```python
from build123d import *

# Parameters (mm, degrees)
F0_W     = 5
F0_H     = 7.5
F2_DEPTH = 39
F3_W     = 41.4538450539
F3_H     = 32
F4_DEPTH = 50
F5_R     = 7.5
F6_DEPTH = 78.001


with BuildPart() as f1:
    # F0 (on Front) → F1 (revolve)
    with BuildSketch(Plane.XZ):
        Polygon((5, 7.5), (5, 0), (19, 0), (19, 3), (35, 3), (35, 7.5), align=None)
        with Locations((2.5, 3.75)):
            Rectangle(F0_W, F0_H)
        Polygon((0, 20), (0, 7.5), (5, 7.5), (5, 30), (0, 30), align=None)
    revolve(axis=Axis((17.5, 0, 0), (1, 0, 0)))

    # F0 (on Front) → F2 (join, symmetric)
    with BuildSketch(Plane.XZ):
        with BuildLine():
            ThreePointArc((-30, -20), (-15.8578643763, -14.1421356237), (-10, 0))
            ThreePointArc((-10, 0), (-15.8578643763, 14.1421356237), (-30, 20))
            ThreePointArc((-30, 20), (-50, 0), (-30, -20))
        make_face()
        with BuildLine():
            Line((-10, 0), (0, 0))
            Line((0, 0), (0, 7.5))
            Line((0, 7.5), (0, 20))
            Line((0, 20), (-30, 20))
            ThreePointArc((-30, 20), (-15.8578643763, 14.1421356237), (-10, 0))
        make_face()
        with BuildLine():
            Line((0, -7.5), (0, 0))
            Line((0, 0), (-10, 0))
            ThreePointArc((-10, 0), (-15.8578643763, -14.1421356237), (-30, -20))
            Line((-30, -20), (0, -20))
            Line((0, -20), (0, -7.5))
        make_face()
    extrude(amount=F2_DEPTH, both=True)

    # F3 (on Top) → F4 (cut, symmetric)
    with BuildSketch(Plane.XY):
        with Locations((-29.273077473, -16)):
            Rectangle(F3_W, F3_H)
        with Locations((-29.273077473, 16)):
            Rectangle(F3_W, F3_H)
    extrude(amount=F4_DEPTH, both=True, mode=Mode.SUBTRACT)

    # F5 (on face) → F6 (cut, through all)
    with BuildSketch(Plane.XZ.offset(39)):
        with Locations((-30, 0)):
            Circle(F5_R)
    extrude(amount=-F6_DEPTH, mode=Mode.SUBTRACT)


solid = f1.part
```
Work out the finished part from the listing and answer in its coordinate system (mm). A direction names the side the tool comes from. Coordinates: 2 decimals unless noted, no trailing zeros. Loops run counter-clockwise (first coordinate to the right, second up) from the corner with the lowest first, then second, coordinate; pieces in that order, holes last. Notation, with made-up numbers: (78.5, 17) -> (132.5, 17) arc R13 ccw to (132.5, 40) -> close; hole circle Ø5 at (-4.75, 85). An arc over 180 degrees is marked (long way). Answer as CSV lines item,"result".
Q1. The part is cut by section D-D on x = 30. Write down the section's boundary in (y, z), and give its area (3 significant figures).
Findings:
outline,"circle Ø15 at (0, 0); hole circle Ø6 at (0, 0)"
area,"148 mm²"
Q2. The part is cut by section A-A on z = 0. Write down the section's boundary in (x, y).
Findings:
outline,"(-50, -39) -> (-37.5, -39) -> (-37.5, -32) -> (-50, -32) -> close; (-50, 32) -> (-37.5, 32) -> (-37.5, 39) -> (-50, 39) -> close; (-22.5, -39) -> (0, -39) -> (0, -30) -> (5, -30) -> (5, -7.5) -> (35, -7.5) -> (35, -3) -> (19, -3) -> (19, 3) -> (35, 3) -> (35, 7.5) -> (5, 7.5) -> (5, 30) -> (0, 30) -> (0, 39) -> (-22.5, 39) -> (-22.5, 32) -> (-8.55, 32) -> (-8.55, -32) -> (-22.5, -32) -> close"
Q3. A tool of negligible diameter and unlimited length cuts with its end or side. For faces 1 (the face through (-5, -1, -20)), 2 (the face through (-8.546, 0, 0)), 3 (the face through (19.79, -0.33, -7.493)), from which of +Z, -Z, +X, -X, +Y, -Y can it reach the whole face along a straight path? Write none if from no direction.
Findings:
face 1,"-Z, -X, +Y, -Y"
face 2,"+Z, -Z, -X"
face 3,"+X"
Q4. Find the intervals of material crossed by probe 1 along Z at (x, y) = (-30, -35.25); probe 2 along Y at (x, z) = (-14.5, -6.5); probe 3 along X at (y, z) = (-18, 0), in increasing order.
Findings:
probe 1,"z = -20 to -7.5, 7.5 to 20"
probe 2,"y = -39 to -32, 32 to 39"
probe 3,"x = -8.55 to 5"
Q5. Each of these flat-tipped pins is pushed along its axis until it touches: pin 1 (5.5 mm diameter, centred on y = 0, z = 0, fed in from -X); pin 2 (13.5 mm diameter, centred on x = -30, z = 0, fed in from -Y); pin 3 (3 mm diameter, centred on y = 0, z = -0.5, fed in from +X); pin 4 (13.5 mm diameter, centred on y = -31.5, z = 4, fed in from +X). Where does it stop, or does it pass through?
Findings:
pin 1,"stops at x = -8.55"
pin 2,"passes through"
pin 3,"stops at x = 19"
pin 4,"stops at x = 5"
Q6. For a pull along Z with two mould halves and no side action, classify faces 4 (the face through (-8, -1, 20)), 5 (the face through (-20, 39, 0)), 6 (the face through (27, 0, -3)) as +Z half, -Z half, draft (parallel to the pull), parting line (faces both ways), or undercut.
Findings:
face 4,"+Z half"
face 5,"draft"
face 6,"undercut"
Q7. The part is cut by section C-C on y = 0. Write down the section's boundary in (x, z), and give its area (3 significant figures).
Findings:
outline,"(-8.55, -20) -> (0, -20) -> (0, -30) -> (5, -30) -> (5, -7.5) -> (35, -7.5) -> (35, -3) -> (19, -3) -> (19, 3) -> (35, 3) -> (35, 7.5) -> (5, 7.5) -> (5, 30) -> (0, 30) -> (0, 20) -> (-8.55, 20) -> close"
area,"996 mm²"
Q8. The part is cut by section B-B on x = -33. Write down the section's boundary in (y, z), and give its area (3 significant figures).
Findings:
outline,"(-39, -19.77) -> (-32, -19.77) -> (-32, -6.87) -> (-39, -6.87) -> close; (-39, 6.87) -> (-32, 6.87) -> (-32, 19.77) -> (-39, 19.77) -> close; (32, -19.77) -> (39, -19.77) -> (39, -6.87) -> (32, -6.87) -> close; (32, 6.87) -> (39, 6.87) -> (39, 19.77) -> (32, 19.77) -> close"
area,"361 mm²"
